Verification items for the finished model (mm, model axes). A direction names the side the tool comes from. Coordinates: 2 decimals unless noted, no trailing zeros. Order: outer loops, then holes, each group sorted by start corner. A loop starts at its lowest first (then second) coordinate and runs counter-clockwise, first axis right, second up. Notation, with made-up numbers: (27, 9) -> (41, 9) arc R8 cw to (41, 22) -> close; hole circle Ø4 at (21, -1). An arc over 180 degrees is marked (long way). Write each question's results on one line, items separated by ' | '. Start each with the question number.
(1) Cross-section at A-A on y = 15. Enter the section's corners in (x, z).
(2) Draft check along X on faces 4 (the flat face through (0, 31, 0)), 5 (the flat face through (-6.45, 8, 0)), 6 (the cylindrical face through (-0.738, 5.07, -2.345)). Enter one of: +X half, -X half, draft (parallel to the pull), parting line (faces both ways), or undercut.
(3) Go/stop test with flat-tipped pins: pin 1 (6 mm diameter, centred on y = 24.5, z = -1, fed in from -X); pin 2 (1 mm diameter, centred on y = 19, z = -3.5, fed in from -X); pin 3 (4 mm diameter, centred on x = -2.5, y = 14.5, fed in from -Z). Record where each tip stops, or that it passes through.
(4) Set-up check for faces 1 (the cylindrical face through (3.695, 21.12, -1.532)), 2 (the flat face through (-7, 4, 0)), 3 (the flat face through (7, 4, 0)): record each of +Z, -Z, +X, -X, +Y, -Y from which the full face is reachable in a straight line by a thin tool's end or side.
(5) Cross-section at B-B on y = 27. Enter the section's corners in (x, z).
Autodesk Inventor part; units mm, degrees
ref_plane "YZ Plane" through (0, 0, 0) normal (1, 0, 0) x (0, 1, 0)
ref_plane "XZ Plane" through (0, 0, 0) normal (0, 1, 0) x (-1, 0, 0)
ref_plane "XY Plane" through (0, 0, 0) normal (0, 0, 1) x (1, 0, 0)
sketch "Sketch1" plane through (0, 0, 0) normal (0, 1, 0) x (-1, 0, 0)
  circle A0 centre (0, 0) radius 7.75
  dimension "d0" = 15.5
extrude "Extrusion1" add sketch "Sketch1" along normal blind 12
sketch "Sketch2" plane through (0, 12, 0) normal (0, 1, 0) x (1, 0, 0)
  circle A0 centre (0, 0) radius 7.75
  circle A1 centre (0, 0) radius 7.75
  line L0 (-6.45, -4.2965) -> (-6.45, 4.2965)
  line L1 (6.45, -4.2965) -> (6.45, 4.2965)
  line L2 (0, -12.5996) -> (0, 16.4995) construction
  dimension "d3" = 12.9
extrude "Extrusion2" cut sketch "Sketch2" against normal blind 8 contours A0 L1 | L0 A0
sketch "Sketch3" plane through (0, 12, 0) normal (0, 1, 0) x (1, 0, 0)
  circle A0 centre (0, 0) radius 4
  dimension "d6" = 8
extrude "Extrusion3" add sketch "Sketch3" along normal blind 19
chamfer "Chamfer1" distance 0.5 angle 45 1 edges at (-4, 31, 0)
thread "Thread1"
chamfer "Chamfer2" distance 0.5 angle 45 3 edges at (0, 12, 7.75) (0, 12, -7.75) (7.75, 0, 0)
sketch "Sketch4" plane through (0, 0, 0) normal (0, -1, 0) x (1, 0, 0)
  point P0 (0, 0)
  point P1 (0, 0)
hole "Hole1" at (0, 0, 0) direction (0, 1, 0) diameter 4.917 depth 10 tip angle 118
sketch "Sketch6" plane through (0, 31, 0) normal (0, 1, 0) x (1, 0, 0)
  circle A0 centre (0, 0) radius 4
  line L0 (2.7, -4) -> (-2.7, -4)
  line L1 (-2.7, -4) -> (-2.7, 4)
  line L2 (-2.7, 4) -> (2.7, 4)
  line L3 (2.7, 4) -> (2.7, -4)
  line L4 (2.7, -4) -> (-2.7, 4) construction
  line L5 (-2.7, -4) -> (2.7, 4) construction
  point P0 (-2.7, -2.9513)
  point P1 (-2.7, 2.9513)
  point P2 (2.7, 2.9513)
  point P3 (2.7, -2.9513)
  dimension "d27" = 5.4
extrude "Extrusion5" cut sketch "Sketch6" against normal blind 5 contours A0 L3 | L1 A0
properties part number "Box Fixing Stud"
Results are:
1) outline: circle Ø8 at (0, 0)
2) face 4: draft | face 5: -X half | face 6: undercut
3) pin 1: stops at x = -4 | pin 2: stops at x = -2.65 | pin 3: stops at z = -3.97
4) face 1: +Y | face 2: +Z, -Z, -X, +Y | face 3: +Z, -Z, +X, +Y
5) outline: (-2.7, -2.95) arc R4 ccw to (2.7, -2.95) -> (2.7, 2.95) arc R4 ccw to (-2.7, 2.95) -> close
